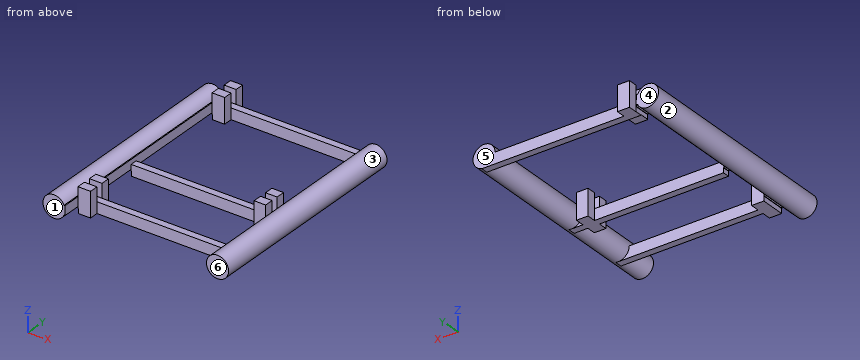
```python
from build123d import *

# Parameters (mm, degrees)
SKETCH2_R             = 2.5
BOSS_EXTRUDE1_DEPTH   = 49.3
BOSS_EXTRUDE1_2_DEPTH = 49.3
BOSS_EXTRUDE2_DEPTH   = 49.3
SKETCH4_W             = 2.5
SKETCH4_H             = 1.56
BOSS_EXTRUDE4_DEPTH   = 35
BOSS_EXTRUDE8_DEPTH   = 2
SKETCH15_W            = 2.621045261
SKETCH15_H            = 5.894157502
BOSS_EXTRUDE10_DEPTH  = 2
SKETCH16_W            = 2.858555501
SKETCH16_H            = 5.670918984
BOSS_EXTRUDE11_DEPTH  = 2
SKETCH17_W            = 2.858555501
SKETCH17_H            = 5.670918984
BOSS_EXTRUDE12_DEPTH  = 2
BOSS_EXTRUDE13_DEPTH  = 2
SKETCH21_W            = 2.718681831
SKETCH21_H            = 5.670918984
BOSS_EXTRUDE16_DEPTH  = 2
SKETCH22_W            = 0.232218322
SKETCH22_H            = 1.447780317
CUT_EXTRUDE3_DEPTH    = 49.4


with BuildPart() as part:
    # Sketch2 → Boss-Extrude1 (new body)
    with BuildSketch(Plane(origin=(0, 0, 0), x_dir=(1, 0, 0), z_dir=(0, 1, 0))):
        with Locations(Location((0, 0, 0), (0, 0, 270))):
            Circle(SKETCH2_R)
    extrude(amount=BOSS_EXTRUDE1_DEPTH)

    # Sketch3 → Boss-Extrude2 (add)
    with BuildSketch(Plane(origin=(0, 0, 0), x_dir=(1, 0, 0), z_dir=(0, 1, 0))):
        with BuildLine():
            Line((2.5, 0), (2.499588142, -0.045377544))
            ThreePointArc((2.499588142, -0.045377544), (2.436264871, -0.560904161), (2.267781678, -1.052219683))
            Line((2.267781678, -1.052219683), (2.267781678, -2.5))
            Line((2.267781678, -2.5), (2.5, -2.5))
            Line((2.5, -2.5), (2.5, 0))
        make_face()
        with BuildLine():
            ThreePointArc((2.267781678, 1.052219683), (2.44125523, 0.538769805), (2.5, 0))
            Line((2.5, 0), (2.5, 2.5))
            Line((2.5, 2.5), (2.267781678, 2.5))
            Line((2.267781678, 2.5), (2.267781678, 1.052219683))
        make_face()
    extrude(amount=BOSS_EXTRUDE2_DEPTH)



with BuildPart() as body_2:
    # Sketch2 → Boss-Extrude1 2 (new body)
    with BuildSketch(Plane(origin=(0, 0, 0), x_dir=(1, 0, 0), z_dir=(0, 1, 0))):
        with Locations(Location((37, 0, 0), (0, 0, 270))):
            Circle(SKETCH2_R)
    extrude(amount=BOSS_EXTRUDE1_2_DEPTH)


with BuildPart() as part_1:
    add(part.part)

    add(body_2.part)  # Boss-Extrude4 merges body 2
    # Sketch4 → Boss-Extrude4 (add)
    with BuildSketch(Plane(origin=(2.5, 0, 0), x_dir=(0, 0, -1), z_dir=(1, 0, 0))):
        with Locations((1.25, 48.52)):
            Rectangle(SKETCH4_W, SKETCH4_H)
        with Locations((1.25, 21.34)):
            Rectangle(SKETCH4_W, SKETCH4_H)
        with Locations((1.25, 6.78)):
            Rectangle(SKETCH4_W, SKETCH4_H)
    extrude(amount=BOSS_EXTRUDE4_DEPTH)

    # Sketch10 → Boss-Extrude8 (add)
    with BuildSketch(Plane(origin=(0, 22.12, 0), x_dir=(1, 0, 0), z_dir=(0, 1, 0))):
        Polygon((31.775974476, 2.5), (31.775974476, -0.65349723), (31.775974476, -2.529631849), (31.775974476, -3.394157502), (34.397019737, -3.394157502), (34.397019737, -2.529631849), (34.397019737, -0.644583093), (34.397019737, 2.5), align=None)
    extrude(amount=BOSS_EXTRUDE8_DEPTH)

    # Sketch15 → Boss-Extrude10 (add)
    with BuildSketch(Plane.XZ.offset(-20.56)):
        with Locations((33.086497107, 0.447078751)):
            Rectangle(SKETCH15_W, SKETCH15_H)
    extrude(amount=BOSS_EXTRUDE10_DEPTH)

    # Sketch16 → Boss-Extrude11 (add)
    with BuildSketch(Plane(origin=(0, 7.56, 0), x_dir=(1, 0, 0), z_dir=(0, 1, 0))):
        with Locations((3.929277751, -0.335459492)):
            Rectangle(SKETCH16_W, SKETCH16_H)
    extrude(amount=BOSS_EXTRUDE11_DEPTH)

    # Sketch17 → Boss-Extrude12 (add)
    with BuildSketch(Plane(origin=(0, 6, 0), x_dir=(-1, 0, 0), z_dir=(0, -1, 0))):
        with Locations((-3.929277751, -0.335459492)):
            Rectangle(SKETCH17_W, SKETCH17_H)
    extrude(amount=BOSS_EXTRUDE12_DEPTH)

    # Sketch18 → Boss-Extrude13 (add)
    with BuildSketch(Plane(origin=(0, 47.74, 0), x_dir=(-1, 0, 0), z_dir=(0, -1, 0))):
        Polygon((-2.5, 2.512386099), (-5.358555501, 2.5), (-5.358555501, -3.170918984), (-2.5, -3.170918984), align=None)
    extrude(amount=BOSS_EXTRUDE13_DEPTH)

    # Sketch21 → Boss-Extrude16 (add)
    with BuildSketch(Plane(origin=(0, 49.3, 0), x_dir=(1, 0, 0), z_dir=(0, 1, 0))):
        with Locations((3.999214586, -0.335459492)):
            Rectangle(SKETCH21_W, SKETCH21_H)
    extrude(amount=BOSS_EXTRUDE16_DEPTH)

    # Sketch22 → Cut-Extrude3 (cut)
    with BuildSketch(Plane(origin=(0, 0, 0), x_dir=(1, 0, 0), z_dir=(0, 1, 0))):
        Polygon((2.267781678, 1.052219683), (2.267781678, 2.5), (2.5, 2.5), (2.593422148, 2.5), (2.593422148, 1.424983609), (2.5, 1.424983609), (2.5, 1.052219683), align=None)
        with Locations((2.383890839, -1.776109842)):
            Rectangle(SKETCH22_W, SKETCH22_H)
    extrude(amount=CUT_EXTRUDE3_DEPTH, mode=Mode.SUBTRACT)


solid = part_1.part
```
Verification items for the finished model (mm, model axes). Face numbers are marked on the shaded views. A direction names the side the tool comes from. Round coordinates to 2 decimals unless told otherwise and drop trailing zeros. Write each loop counter-clockwise with the first axis right and the second up, starting at its lowest first coordinate (ties: lowest second). Pieces come first, ordered by that corner, then holes. Notation, with made-up numbers: (-4, -6) -> (44, -6) arc R18 cw to (44, 0) -> close; hole circle Ø8 at (78.25, 44.5). An arc over 180 degrees is marked (long way). Write each question's results on one line, items separated by ' | '. Start each with the question number.
1. Material ranges on probe 1 along Y at (x, z) = (28, -1.45); probe 2 along Y at (x, z) = (34, -0.55); probe 3 along X at (y, z) = (35.5, 0.15), recorded low to high. Write a range as from..to.
2. Set-up check for the marked faces 4, 5 and 6: record each of +Z, -Z, +X, -X, +Y, -Y from which the full face is reachable in a straight line by a thin tool's end or side.
3. Cross-section at A-A (x = 8). Enter the section's corners in (y, z), then the cut area to 3 significant figures.
4. Depth check by flat-ended pin: P1, Ø1.7, axis at x = 21.5, y = 6.5, coming from the +Z side; P2, Ø3, axis at x = 14, y = 6, coming from the -Z side; P3, Ø1.3, axis at x = 36, z = -1, coming from the +Y side. Enter the tip coordinate at first touch or a pass-through.
5. Cross-section at C-C (z = 1.95). Count the separate pieces of the cut face and the enclosed holes in it, then the cut area to 3 significant figures.
6. Cross-section at B-B (y = 12.5). Enter the section's corners in (x, z), then the cut area to 3 significant figures.
7. Cross-section at D-D (x = 0). Enter the section's corners in (y, z).
8. Draft check along X on the marked faces 1, 2 and 3. Enter one of: +X half, -X half, draft (parallel to the pull), parting line (faces both ways), or undercut.
Solutions:
1) probe 1: y = 6..7.56, 20.56..22.12, 47.74..49.3 | probe 2: y = 6..7.56, 18.56..24.12, 47.74..49.3 | probe 3: x = -2.5..2.5, 34.5..39.5
2) face 4: +Z, -Z, -X, +Y | face 5: +Z, -Z, +X, +Y | face 6: +Z, -Z, +X, -X, -Y
3) outline: (6, -2.5) -> (7.56, -2.5) -> (7.56, 0) -> (6, 0) -> close; (20.56, -2.5) -> (22.12, -2.5) -> (22.12, 0) -> (20.56, 0) -> close; (47.74, -2.5) -> (49.3, -2.5) -> (49.3, 0) -> (47.74, 0) -> close | area: 11.7 mm2
4) P1: stops at z = 0 | P2: stops at z = -2.5 | P3: stops at y = 49.3
5) separate pieces: 8 | enclosed holes: 0 | area: 342 mm2
6) outline: (2.27, -1.05) -> (2.5, -1.05) -> (2.5, 1.05) -> (2.27, 1.05) arc R2.5 ccw (long way) to start; circle Ø5 at (37, 0) | area: 39.4 mm2
7) outline: (0, -2.5) -> (49.3, -2.5) -> (49.3, 2.5) -> (0, 2.5) -> close
8) face 1: draft | face 2: undercut | face 3: undercut
